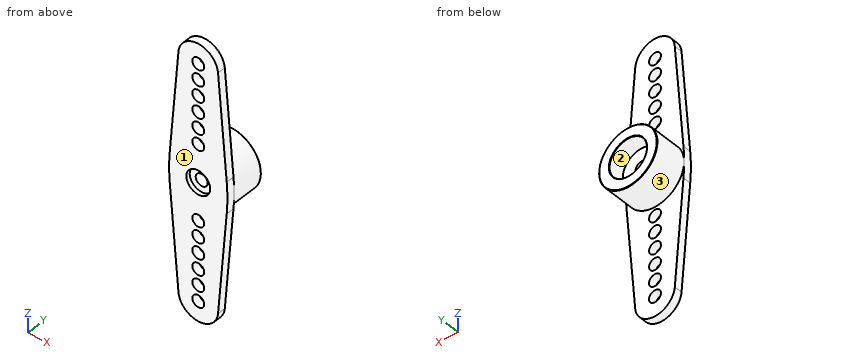
from build123d import *

# Parameters (mm, degrees)
SKETCH1_R           = 0.75
BOSS_EXTRUDE1_DEPTH = 1
SKETCH2_R           = 3.666938222
SKETCH2_R_2         = 1.5
SKETCH2_R_3         = 0.75
BOSS_EXTRUDE2_DEPTH = 5
SKETCH2_2_R         = 1.5
CUT_EXTRUDE1_DEPTH  = 0.5
SKETCH3_R           = 2.355
CUT_EXTRUDE2_DEPTH  = 2
CHAMFER1_SIZE       = 0.05


with BuildPart() as part:
    # Sketch1 → Boss-Extrude1 (new body)
    with BuildSketch(Plane(origin=(0, 0, 0), x_dir=(1, 0, 0), z_dir=(0, 1, 0))):
        with BuildLine():
            Line((-2.49119588, 14.959626071), (-3.584168958, 1.970735827))
            ThreePointArc((-3.584168958, 1.970735827), (-3.666938222, 0), (-3.584168958, -1.970735827))
            Line((-3.584168958, -1.970735827), (-2.49119588, -14.959626071))
            ThreePointArc((-2.49119588, -14.959626071), (0, -17.25), (2.49119588, -14.959626071))
            Line((2.49119588, -14.959626071), (3.584168958, -1.970735827))
            ThreePointArc((3.584168958, -1.970735827), (3.666938222, 0), (3.584168958, 1.970735827))
            Line((3.584168958, 1.970735827), (2.49119588, 14.959626071))
            ThreePointArc((2.49119588, 14.959626071), (0, 17.25), (-2.49119588, 14.959626071))
        make_face()
        with Locations(Location((0, 14.75, 0), (0, 0, 270))):
            Circle(SKETCH1_R, mode=Mode.SUBTRACT)
        with Locations(Location((0, 12.75, 0), (0, 0, 270))):
            Circle(SKETCH1_R, mode=Mode.SUBTRACT)
        with Locations(Location((0, 10.75, 0), (0, 0, 270))):
            Circle(SKETCH1_R, mode=Mode.SUBTRACT)
        with Locations(Location((0, 8.75, 0), (0, 0, 270))):
            Circle(SKETCH1_R, mode=Mode.SUBTRACT)
        with Locations(Location((0, 6.75, 0), (0, 0, 270))):
            Circle(SKETCH1_R, mode=Mode.SUBTRACT)
        with Locations(Location((0, 4.75, 0), (0, 0, 270))):
            Circle(SKETCH1_R, mode=Mode.SUBTRACT)
        with Locations(Location((0, 0, 0), (0, 0, 270))):
            Circle(SKETCH1_R, mode=Mode.SUBTRACT)
        with Locations(Location((0, -14.75, 0), (0, 0, 90))):
            Circle(SKETCH1_R, mode=Mode.SUBTRACT)
        with Locations(Location((0, -12.75, 0), (0, 0, 90))):
            Circle(SKETCH1_R, mode=Mode.SUBTRACT)
        with Locations(Location((0, -10.75, 0), (0, 0, 90))):
            Circle(SKETCH1_R, mode=Mode.SUBTRACT)
        with Locations(Location((0, -8.75, 0), (0, 0, 90))):
            Circle(SKETCH1_R, mode=Mode.SUBTRACT)
        with Locations(Location((0, -6.75, 0), (0, 0, 90))):
            Circle(SKETCH1_R, mode=Mode.SUBTRACT)
        with Locations(Location((0, -4.75, 0), (0, 0, 90))):
            Circle(SKETCH1_R, mode=Mode.SUBTRACT)
    extrude(amount=BOSS_EXTRUDE1_DEPTH)

    # Sketch2 → Boss-Extrude2 (add)
    with BuildSketch(Plane.XZ):
        with Locations(Location((0, 0, 0), (0, 0, 270))):
            Circle(SKETCH2_R)
        Circle(SKETCH2_R_2, mode=Mode.SUBTRACT)
        Circle(SKETCH2_R_2)
        with Locations(Location((0, 0, 0), (0, 0, 270))):
            Circle(SKETCH2_R_3, mode=Mode.SUBTRACT)
    extrude(amount=-BOSS_EXTRUDE2_DEPTH)

    # Sketch2_2 → Cut-Extrude1 (cut)
    with BuildSketch(Plane.XZ):
        with Locations(Location((0, 0, 0), (0, 0, 270))):
            Circle(SKETCH2_2_R)
    extrude(amount=-CUT_EXTRUDE1_DEPTH, mode=Mode.SUBTRACT)

    # Sketch3 → Cut-Extrude2 (cut)
    with BuildSketch(Plane(origin=(0, 5, 0), x_dir=(1, 0, 0), z_dir=(0, 1, 0))):
        with Locations(Location((0, 0, 0), (0, 0, 270))):
            Circle(SKETCH3_R)
    extrude(amount=-CUT_EXTRUDE2_DEPTH, mode=Mode.SUBTRACT)

    # Chamfer1
    chamfer1_edges = [part.edges().sort_by_distance(p)[0] for p in [
        (0, 5, 3.666938222),
        (0, 5, -2.355),
    ]]
    chamfer(chamfer1_edges, length=CHAMFER1_SIZE)


solid = part.part
Check sheet for the modelled part. Datum: model origin and axes. Units: mm. Face numbers are marked on the shaded views. Give positions to 0.01 mm unless a question says otherwise; leave off trailing zeros. Loops run counter-clockwise (first coordinate to the right, second up) from the corner with the lowest first, then second, coordinate; pieces in that order, holes last. Notation, with made-up numbers: M 38.5,82.5 L 81.5,82.5 A21 cw 81.5,119.5 Z; hole C 89.25,62 d2. An arc over 180 degrees is marked long. Use a Markdown table: item, result. Add a question column.
Q1. Sectioned sample at C-C, the plane x = 0. Give the number of separate pieces and of enclosed holes in the cut face, then the cut area to 3 significant figures.
Q2. Sectioned sample at B-B, the plane y = 1.9. Record the cut outline in (x, z).
Q3. Sectioned sample at A-A, the plane z = 5. Record the cut outline in (x, y), then the cut area to 3 significant figures.
Q4. Go/stop test with flat-tipped pins: pin 1 (1 mm diameter, centred on x = -3, z = -12.5, fed in from +Y); pin 2 (0.9 mm diameter, centred on x = 0, z = 14.75, fed in from +Y); pin 3 (1.5 mm diameter, centred on x = -1, y = 2.5, fed in from +Z). Record where each tip stops, or that it passes through.
Q5. Scan lines: line 1 along Y through (x, z) = (-1.75, 15); line 2 along X through (y, z) = (0.7, 8.75); line 3 along X through (y, z) = (0.5, 14.75). Record each from-to range of solid material in increasing order. Write a range as [from, to].
Q6. Sectioned sample at D-D, the plane z = 10.75. Record the cut outline in (x, y).
Q7. Mould release check, pull along X, two halves, no side actions. Record for the marked faces 1, 2 and 3: pulls with the +X half, pulls with the -X half, needs draft (parallel to the pull), parting line crosses it, or undercut.
Verdict:
| question | item | result |
|---|---|---|
| 1 | separate pieces | 14 |
| 1 | enclosed holes | 0 |
| 1 | area | 31.2 mm^2 |
| 2 | outline | C 0,0 d7.33; hole C 0,0 d1.5 |
| 3 | outline | M -3.33,0 L -0.71,0 L -0.71,1 L -3.33,1 Z; M 0.71,0 L 3.33,0 L 3.33,1 L 0.71,1 Z |
| 3 | area | 5.24 mm^2 |
| 4 | pin 1 | y = 1 |
| 4 | pin 2 | through |
| 4 | pin 3 | z = 3.66 |
| 5 | line 1 | [0, 1] |
| 5 | line 2 | [-3.01, -0.75], [0.75, 3.01] |
| 5 | line 3 | [-2.51, -0.75], [0.75, 2.51] |
| 6 | outline | M -2.85,0 L -0.75,0 L -0.75,1 L -2.85,1 Z; M 0.75,0 L 2.85,0 L 2.85,1 L 0.75,1 Z |
| 7 | face 1 | needs draft |
| 7 | face 2 | undercut |
| 7 | face 3 | parting line crosses it |
